Geometry: final body of the model. Coordinates: model frame, mm. Face numbers are marked on the shaded views. A direction names the side the tool comes from. Give positions to 0.01 mm unless a question says otherwise; leave off trailing zeros. Write each loop counter-clockwise with the first axis right and the second up, starting at its lowest first coordinate (ties: lowest second). Pieces come first, ordered by that corner, then holes. Notation, with made-up numbers: (37, 44.25) - (87, 44.25) arc R22 ccw to (87, 55.25) - close; hole circle Ø1 at (-18, -5.75). An arc over 180 degrees is marked (long way). Return JSON: item names as keys, results as strings.
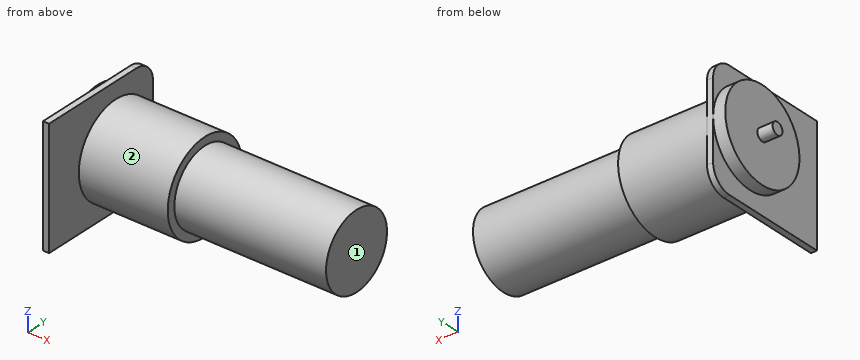
from build123d import *

# Parameters (mm, degrees)
BOSS_EXTRUDE1_DEPTH = 3
SKETCH2_R           = 22.5
BOSS_EXTRUDE2_DEPTH = 44
SKETCH3_R           = 18.5
BOSS_EXTRUDE3_DEPTH = 75
SKETCH4_R           = 22.5
BOSS_EXTRUDE4_DEPTH = 6
SKETCH5_R           = 3
BOSS_EXTRUDE5_DEPTH = 7.5


with BuildPart() as part:
    # Sketch1 → Boss-Extrude1 (new body)
    with BuildSketch(Plane(origin=(0, 0, 0), x_dir=(0, 0, -1), z_dir=(1, 0, 0))):
        with BuildLine():
            Line((-10, -1.222482436), (-48, -1.222482436))
            ThreePointArc((-48, -1.222482436), (-55.071067812, -4.151414624), (-58, -11.222482436))
            Line((-58, -11.222482436), (-58, -64.222482436))
            Line((-58, -64.222482436), (0, -64.222482436))
            Line((0, -64.222482436), (0, -11.222482436))
            ThreePointArc((0, -11.222482436), (-2.928932188, -4.151414624), (-10, -1.222482436))
        make_face()
    extrude(amount=BOSS_EXTRUDE1_DEPTH)

    # Sketch2 → Boss-Extrude2 (add)
    with BuildSketch(Plane(origin=(3, 0, 0), x_dir=(0, 0, -1), z_dir=(1, 0, 0))):
        with Locations(Location((-27.5, -23.722482436, 0), (0, 0, 90))):
            Circle(SKETCH2_R)
    extrude(amount=BOSS_EXTRUDE2_DEPTH)

    # Sketch3 → Boss-Extrude3 (add)
    with BuildSketch(Plane(origin=(47, 0, 0), x_dir=(0, 0, -1), z_dir=(1, 0, 0))):
        with Locations((-27.5, -23.722482436)):
            Circle(SKETCH3_R)
    extrude(amount=BOSS_EXTRUDE3_DEPTH)

    # Sketch4 → Boss-Extrude4 (add)
    with BuildSketch(Plane.ZY):
        with Locations(Location((30.5, -23.722482436, 0), (0, 0, 90))):
            Circle(SKETCH4_R)
    extrude(amount=BOSS_EXTRUDE4_DEPTH)

    # Sketch5 → Boss-Extrude5 (add)
    with BuildSketch(Plane.ZY.offset(6)):
        with Locations((30.5, -23.722482436)):
            Circle(SKETCH5_R)
    extrude(amount=BOSS_EXTRUDE5_DEPTH)


solid = part.part
Q1. Pin query (flat end, axial travel): P1, Ø8, axis at x = 16.5, y = -14, coming from the -Z side; P2, Ø1.5, axis at y = -32.5, z = 14, coming from the -X side; P3, Ø5, axis at y = -55.5, z = 17.5, coming from the +X side. Return the tip coordinate at first contact, or that it passes through.
Answer key:
{"P1": "stops at z = 5.74", "P2": "stops at x = -6", "P3": "stops at x = 3"}
Q2. Set-up query: the marked faces 1 and 2. Return all of +Z, -Z, +X, -X, +Y, -Y with unobstructed straight access to the full face (end or side cutting, diameter ignored); none if empty.
Answer key:
{"face 1": "+Z, -Z, +X, +Y, -Y", "face 2": "+X"}
Q3. Section query A-A, the plane y = -13. Return the cut outline in (x, z), plus the area to 3 significant figures.
Answer key:
{"outline": "(-6, 10.72) - (0, 10.72) - (0, 0) - (3, 0) - (3, 7.72) - (47, 7.72) - (47, 12.42) - (122, 12.42) - (122, 42.58) - (47, 42.58) - (47, 47.28) - (3, 47.28) - (3, 58) - (0, 58) - (0, 50.28) - (-6, 50.28) - close", "area": "4,410 mm^2"}
Q4. Section query D-D, the plane x = 89. Return the cut outline in (y, z).
Answer key:
{"outline": "circle Ø37 at (-23.72, 27.5)"}
Q5. Section query B-B, the plane z = 43. Return the cut outline in (x, y).
Answer key:
{"outline": "(-6, -42.43) - (0, -42.43) - (0, -64.22) - (3, -64.22) - (3, -40.03) - (47, -40.03) - (47, -33.82) - (122, -33.82) - (122, -13.62) - (47, -13.62) - (47, -7.41) - (3, -7.41) - (3, -1.22) - (0, -1.22) - (0, -5.01) - (-6, -5.01) - close"}
Q6. Material intervals for probe 1 along X at (y, z) = (-13, 9.5); probe 2 along Z at (x, y) = (84.5, -24); probe 3 along X at (y, z) = (-33.5, 52), sorted ascending. Write a range as [from, to].
Answer key:
{"probe 1": "x = [0, 47]", "probe 2": "z = [9, 46]", "probe 3": "x = [0, 3]"}
Q7. Section query C-C, the plane x = -4. Return the cut outline in (y, z).
Answer key:
{"outline": "circle Ø45 at (-23.72, 30.5)"}
